Could you check a few things on this drawing? It's one solid part, dimensions in mm from its lowest x, y, z. Give positions to 0.01 mm unless a question says otherwise; leave off trailing zeros. Write each loop counter-clockwise with the first axis right and the second up, starting at its lowest first coordinate (ties: lowest second). Pieces come first, ordered by that corner, then holes. Notation, with made-up numbers: M 81,2.5 L 116,2.5 A15 cw 116,26.5 Z; hole C -12,1.5 d7. An arc over 180 degrees is marked long. Answer as CSV lines item,"result". Start each with the question number.
Q1. Suppose I cut it at A-A (y = 43). Write out the boundary of the cut face in (x, z).
Q2. Suppose I cut it at B-B (x = 22.5). Write out the boundary of the cut face in (y, z), then the cut area to 3 significant figures.
Q3. If I drill on line 1 along X through (y, z) = (28, 0.5); line 2 along Y through (x, z) = (22.5, 0.55); line 3 along Y through (x, z) = (18.5, 0.15), over which ranges is the centre line in solid material (lowest first)?
Q4. For pin 1 (5 mm diameter, centred on x = 22.5, y = 7.5, fed in from -Z); pin 2 (1 mm diameter, centred on x = 22, z = 1, fed in from +Y); pin 3 (0.6 mm diameter, centred on x = 4, z = 1, fed in from -Y), each with a flat end and sliding along its axis, tell me the tip position at first contact or that it passes through.
Q5. Suppose I cut it at D-D (z = 0.6). Write out the boundary of the cut face in (x, y).
Q6. Suppose I cut it at C-C (y = 7.5). Write out the boundary of the cut face in (x, z), then the cut area to 3 significant figures.
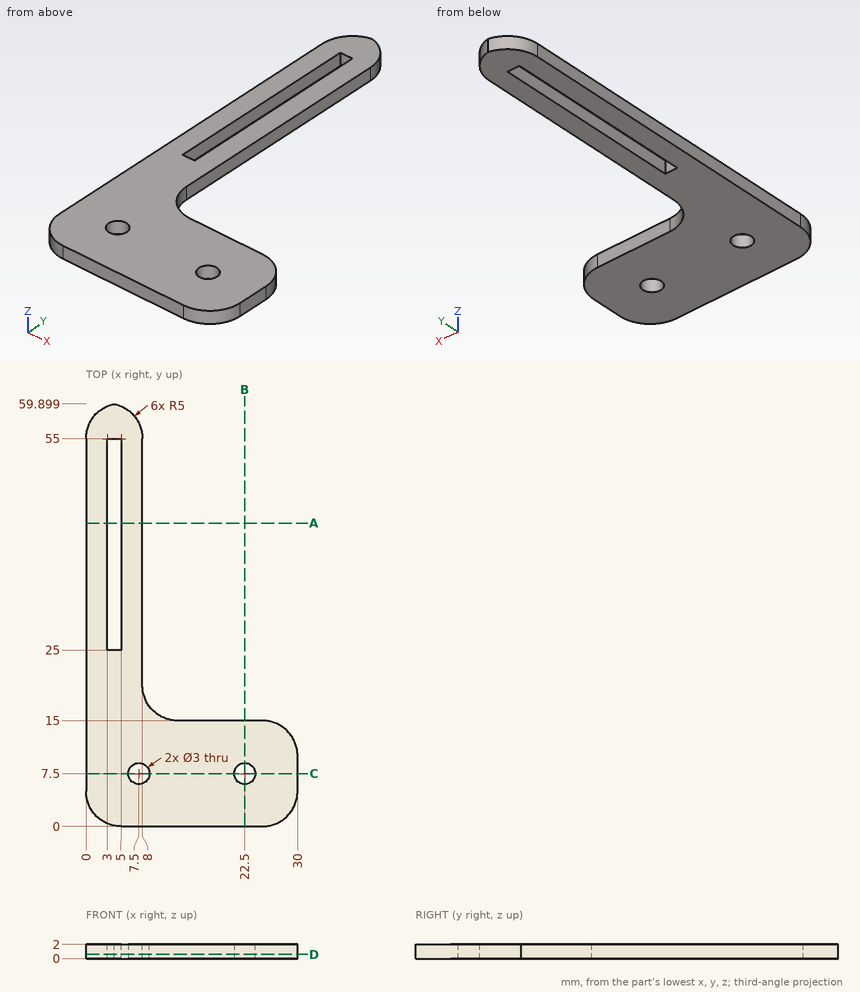
Resolved:
1,outline,"M 0,0 L 3,0 L 3,2 L 0,2 Z; M 5,0 L 8,0 L 8,2 L 5,2 Z"
2,outline,"M 0,0 L 6,0 L 6,2 L 0,2 Z; M 9,0 L 15,0 L 15,2 L 9,2 Z"
2,area,"24.0 mm^2"
3,line 1,"0 to 3, 5 to 8"
3,line 2,"0 to 6, 9 to 15"
3,line 3,"0 to 15"
4,pin 1,"z = 0"
4,pin 2,"y = 15"
4,pin 3,"y = 0.05"
5,outline,"M 0,5 A5 ccw 5,0 L 25,0 A5 ccw 30,5 L 30,10 A5 ccw 25,15 L 13,15 A5 cw 8,20 L 8,55 A5 ccw 4,59.9 A5 ccw 0,55 Z; hole M 3,25 L 5,25 L 5,55 L 3,55 Z; hole C 7.5,7.5 d3; hole C 22.5,7.5 d3"
6,outline,"M 0,0 L 6,0 L 6,2 L 0,2 Z; M 9,0 L 21,0 L 21,2 L 9,2 Z; M 24,0 L 30,0 L 30,2 L 24,2 Z"
6,area,"48.0 mm^2"
